```python
from build123d import *

# Parameters (mm, degrees)
SKETCH1_W                = 34
SKETCH1_H                = 46.5
BOSS_EXTRUDE1_DEPTH      = 28.5
SKETCH2_R                = 1.45
CUT_EXTRUDE1_DEPTH       = 51.088047476
SKETCH3_W                = 28.5
SKETCH3_H                = 20
CUT_EXTRUDE2_DEPTH       = 51.088047476
SKETCH4_W                = 26
SKETCH4_H                = 20
CUT_EXTRUDE3_DEPTH       = 41.519285532
BOSS_EXTRUDE2_DEPTH      = 5
BOSS_EXTRUDE2_DEPTH_BACK = 3
SKETCH5_W                = 7.437082776
SKETCH5_H                = 15
BOSS_EXTRUDE3_START      = 5.6
SKETCH6_W                = 28.5
SKETCH6_H                = 20
SKETCH6_R                = 1.45
BOSS_EXTRUDE3_DEPTH      = 5.6
SKETCH7_W                = 5.6
SKETCH7_H                = 26.5
CUT_EXTRUDE4_DEPTH       = 43.858050586
SKETCH9_W                = 7.1
SKETCH9_H                = 14
SKETCH9_H_2              = 16.896851025
BOSS_EXTRUDE4_DEPTH      = 4
SKETCH10_W               = 7.1
SKETCH10_H               = 17
BOSS_EXTRUDE5_DEPTH      = 1
SKETCH11_W               = 7.1
SKETCH11_H               = 19
BOSS_EXTRUDE6_DEPTH      = 2
SKETCH12_W               = 7.1
SKETCH12_H               = 16.896851025
BOSS_EXTRUDE7_DEPTH      = 1
CUT_EXTRUDE5_DEPTH       = 47.469048839
CUT_EXTRUDE5_DEPTH_BACK  = 47.469048839
SKETCH13_W               = 7.437082776
SKETCH13_H               = 3
FILLET1_R                = 5
CHAMFER1_START           = -11.4
CHAMFER1_DEPTH           = 25.4
CHAMFER1_START_2         = 9.9
CHAMFER1_2_DEPTH         = 12.1
CHAMFER1_3_DEPTH         = 14.2


with BuildPart() as part:
    # Sketch1 → Boss-Extrude1 (new body)
    with BuildSketch(Plane.XY):
        Rectangle(SKETCH1_W, SKETCH1_H)
    extrude(amount=BOSS_EXTRUDE1_DEPTH)

    # Sketch2 → Cut-Extrude1 (cut, through all)
    with BuildSketch(Plane(origin=(17, 0, 0), x_dir=(0, 0, -1), z_dir=(1, 0, 0))):
        with Locations(Location((-25.25, 20, 0), (0, 0, 90))):
            Circle(SKETCH2_R)
        with Locations(Location((-3.25, 20, 0), (0, 0, 90))):
            Circle(SKETCH2_R)
        with Locations(Location((-3.25, -20, 0), (0, 0, 90))):
            Circle(SKETCH2_R)
        with Locations(Location((-25.25, -20, 0), (0, 0, 90))):
            Circle(SKETCH2_R)
    extrude(amount=-CUT_EXTRUDE1_DEPTH, mode=Mode.SUBTRACT)

    # Sketch3 → Cut-Extrude2 (cut, through all)
    with BuildSketch(Plane(origin=(17, 0, 0), x_dir=(0, 0, -1), z_dir=(1, 0, 0))):
        with Locations((-14.25, -13.25)):
            Rectangle(SKETCH3_W, SKETCH3_H)
    extrude(amount=-CUT_EXTRUDE2_DEPTH, mode=Mode.SUBTRACT)

    # Sketch4 → Cut-Extrude3 (cut, through all)
    with BuildSketch(Plane(origin=(0, 0, 0), x_dir=(-1, 0, 0), z_dir=(0, 0, -1))):
        with Locations((0, 13.25)):
            Rectangle(SKETCH4_W, SKETCH4_H)
    extrude(amount=-CUT_EXTRUDE3_DEPTH, mode=Mode.SUBTRACT)

    # Sketch5 → Boss-Extrude2 (add, two sides: drawn at the far end of the back side and taken through both)
    with BuildSketch(Plane(origin=(17, 0, 0), x_dir=(0, 0, -1), z_dir=(1, 0, 0)).offset(-BOSS_EXTRUDE2_DEPTH_BACK)):
        with Locations((-3.718541388, -2.75)):
            Rectangle(SKETCH5_W, SKETCH5_H)
    extrude(amount=BOSS_EXTRUDE2_DEPTH + BOSS_EXTRUDE2_DEPTH_BACK)

    # Sketch6 → Boss-Extrude3 (add)
    with BuildSketch(Plane(origin=(-13, 0, 0), x_dir=(0, 0, -1), z_dir=(1, 0, 0)).offset(BOSS_EXTRUDE3_START)):
        with Locations((-14.25, 13.25)):
            Rectangle(SKETCH6_W, SKETCH6_H)
        with Locations(Location((-25.25, 20, 0), (0, 0, 90))):
            Circle(SKETCH6_R, mode=Mode.SUBTRACT)
        with Locations(Location((-3.25, 20, 0), (0, 0, 90))):
            Circle(SKETCH6_R, mode=Mode.SUBTRACT)
    extrude(amount=-BOSS_EXTRUDE3_DEPTH)

    # Sketch7 → Cut-Extrude4 (cut, through all)
    with BuildSketch(Plane(origin=(0, 0, 0), x_dir=(-1, 0, 0), z_dir=(0, 0, -1))):
        with Locations((14.2, 10)):
            Rectangle(SKETCH7_W, SKETCH7_H)
    extrude(amount=-CUT_EXTRUDE4_DEPTH, mode=Mode.SUBTRACT)

    # Sketch9 → Boss-Extrude4 (add)
    with BuildSketch(Plane.XZ.offset(3.25)):
        with Locations((-7.85, 21.5)):
            Rectangle(SKETCH9_W, SKETCH9_H)
        Polygon((2.8, 28.5), (-4.3, 28.5), (-4.3, 14.5), (-4.3, 11.5), (2.8, 11.5), align=None)
        with Locations((13.45, 20.051574487)):
            Rectangle(SKETCH9_W, SKETCH9_H_2)
        Polygon((9.9, 28.5), (2.8, 28.5), (2.8, 11.5), (2.8, 9.5), (9.9, 9.5), (9.9, 11.603148975), align=None)
    extrude(amount=BOSS_EXTRUDE4_DEPTH)

    # Sketch10 → Boss-Extrude5 (add)
    with BuildSketch(Plane.XZ.offset(7.25)):
        with Locations((-0.75, 20)):
            Rectangle(SKETCH10_W, SKETCH10_H)
    extrude(amount=BOSS_EXTRUDE5_DEPTH)

    # Sketch11 → Boss-Extrude6 (add)
    with BuildSketch(Plane.XZ.offset(7.25)):
        with Locations((6.35, 19)):
            Rectangle(SKETCH11_W, SKETCH11_H)
    extrude(amount=BOSS_EXTRUDE6_DEPTH)

    # Sketch12 → Boss-Extrude7 (add)
    with BuildSketch(Plane.XZ.offset(7.25)):
        with Locations((13.45, 20.051574487)):
            Rectangle(SKETCH12_W, SKETCH12_H)
    extrude(amount=BOSS_EXTRUDE7_DEPTH)

    # Sketch13 → Cut-Extrude5 (cut, two sides: drawn at the far end of the back side and taken through both)
    with BuildSketch(Plane(origin=(17, 0, 0), x_dir=(0, 0, -1), z_dir=(1, 0, 0)).offset(-CUT_EXTRUDE5_DEPTH_BACK)):
        Polygon((-19, -9.25), (-28.5, 7.5), (-28.5, -9.25), align=None)
        with Locations((-3.718541388, -8.75)):
            Rectangle(SKETCH13_W, SKETCH13_H)
    extrude(amount=CUT_EXTRUDE5_DEPTH + CUT_EXTRUDE5_DEPTH_BACK, mode=Mode.SUBTRACT)

    # Fillet1
    fillet1_edges = [part.edges().sort_by_distance(p)[0] for p in [
        (22, -7.25, 3.718541388),
    ]]
    fillet(fillet1_edges, radius=FILLET1_R)

    # Chamfer1: read off the stored shape, not the designer's step
    # Chamfer1 outline → Chamfer1 (cut)
    with BuildSketch(Plane.YZ.offset(CHAMFER1_START)):
        Polygon((-2.75, 9.5), (-3.25, 9.5), (-3.25, 0), (6.75, 0), align=None)
    extrude(amount=CHAMFER1_DEPTH, mode=Mode.SUBTRACT)

    # Chamfer1 2 outline → Chamfer1 2 (cut)
    with BuildSketch(Plane.YZ.offset(CHAMFER1_START_2)):
        Polygon((-3.25, 7.437082776), (-0.687082776, 7.437082776), (-3.25, 10), align=None)
    extrude(amount=CHAMFER1_2_DEPTH, mode=Mode.SUBTRACT)

    # Chamfer1 3 outline → Chamfer1 3 (cut)
    with BuildSketch(Plane.YZ.offset(CHAMFER1_START)):
        Polygon((-3.25, 9.5), (-2.75, 9.5), (-3.25, 10), align=None)
    extrude(amount=CHAMFER1_3_DEPTH, mode=Mode.SUBTRACT)


solid = part.part
```
The model under review builds one solid part; all positions refer to its coordinate system, in mm. A direction names the side the tool comes from. Round coordinates to 2 decimals unless told otherwise and drop trailing zeros. Write each loop counter-clockwise with the first axis right and the second up, starting at its lowest first coordinate (ties: lowest second). Pieces come first, ordered by that corner, then holes. Notation, with made-up numbers: (64.5, 52) - (70.5, 52) arc R14 cw to (70.5, 61) - close; hole circle Ø8 at (-0.5, 5.5). An arc over 180 degrees is marked (long way). Answer as CSV lines item,"result". Start each with the question number.
(1) Draft analysis for pull direction X (two halves, no side actions). For faces 4 (the flat face through (13, 13, 14)), 5 (the flat face through (3, 3.25, 15)), 6 (the flat face through (6, -6, 9.5)), 7 (the flat face through (-11.4, 12, 14)), state which applies: pulls with the +X half, pulls with the -X half, needs draft (parallel to the pull), parting line crosses it, or undercut.
(2) We need section B-B on z = 25.25. State the section outline as (x, y) points.
(3) For faces 1 (the flat face through (13, -3.25, 11)), 2 (the flat face through (-1, -8.25, 16)), 3 (the flat face through (13, -8.25, 16)), list the 3-axis set-ups (+Z, -Z, +X, -X, +Y, -Y) from which the entire face can be reached by the end or side of a thin tool; tool diameter is ignored.
(4) For pin 1 Ø6.5 at (x, y) = (16.5, -1.5) entering from +Z; pin 2 Ø3.5 at (y, z) = (0, 2.5) entering from -X; pin 3 Ø12 at (x, z) = (4.5, 18) entering from +Y; pin 4 Ø2.5 at (y, z) = (20, 25.25) entering from -X, all flat-tipped, find the tip position at first contact; note any pin that passes through.
(5) We need section C-C on z = 14. State the section outline as (x, y) points, plus the area to 3 significant figures.
(6) To check wall thickness, follow line 1 (Z direction, x = 14, y = 20); line 2 (X direction, y = 19.5, z = 6); line 3 (X direction, y = -3.5, z = 11.75). State the ranges of each line that lie inside material, in increasing order.
(7) We need section D-D on x = 5. State the section outline as (y, z) points.
(8) We need section A-A on y = 19. State the section outline as (x, z) points.
Worked answers:
1,face 4,"undercut"
1,face 5,"undercut"
1,face 6,"needs draft"
1,face 7,"pulls with the -X half"
2,outline,"(-11.4, 1.77) - (17, 1.77) - (17, 18.55) - (13, 18.55) - (13, 3.25) - (-7.4, 3.25) - (-7.4, 18.55) - (-11.4, 18.55) - close; (-11.4, 21.45) - (-7.4, 21.45) - (-7.4, 23.25) - (-11.4, 23.25) - close; (13, 21.45) - (17, 21.45) - (17, 23.25) - (13, 23.25) - close"
3,face 1,"+X, -Y"
3,face 2,"+Z, -Z, -X, -Y"
3,face 3,"+Z, -Z, +X, -Y"
4,pin 1,"z = 25.24"
4,pin 2,"x = 14"
4,pin 3,"y = 3.25"
4,pin 4,"through"
5,outline,"(-11.4, -3.25) - (-4.3, -3.25) - (-4.3, -8.25) - (2.8, -8.25) - (2.8, -9.25) - (9.9, -9.25) - (9.9, -8.25) - (17, -8.25) - (17, 23.25) - (13, 23.25) - (13, 3.25) - (-7.4, 3.25) - (-7.4, 23.25) - (-11.4, 23.25) - close"
5,area,"458 mm²"
6,line 1,"0 to 1.8, 4.7 to 23.8, 26.7 to 28.5"
6,line 2,"-11.4 to -7.4, 13 to 17"
6,line 3,"-4.3 to 17"
7,outline,"(-9.25, 9.5) - (-2.75, 9.5) - (3.25, 3.5) - (3.25, 26.09) - (-9.25, 19) - close"
8,outline,"(-11.4, 0) - (-7.4, 0) - (-7.4, 2.2) - (-11.4, 2.2) - close; (-11.4, 4.3) - (-7.4, 4.3) - (-7.4, 24.2) - (-11.4, 24.2) - close; (-11.4, 26.3) - (-7.4, 26.3) - (-7.4, 28.5) - (-11.4, 28.5) - close; (13, 0) - (17, 0) - (17, 2.2) - (13, 2.2) - close; (13, 4.3) - (17, 4.3) - (17, 24.2) - (13, 24.2) - close; (13, 26.3) - (17, 26.3) - (17, 28.5) - (13, 28.5) - close"
